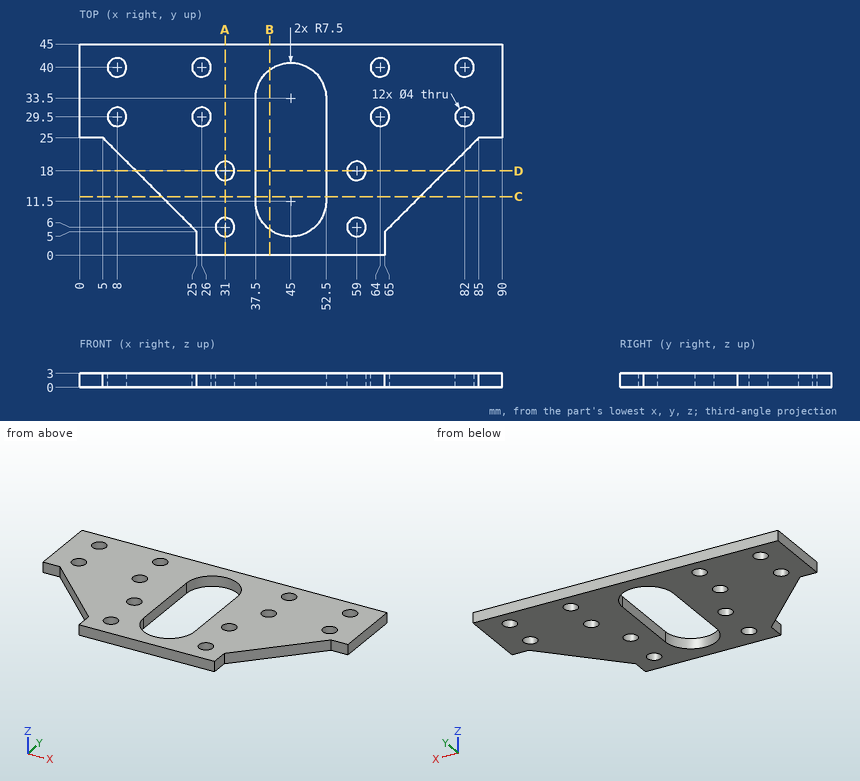
Part print with two shaded views. Sizes in mm from the minimum x, y, z corner. Coordinates: 2 decimals unless noted, no trailing zeros. Order: outer loops, then holes, each group sorted by start corner. A loop starts at its lowest first (then second) coordinate and runs counter-clockwise, first axis right, second up. Notation, with made-up numbers: (-21, 76.5) - (5, 76.5) arc R8 ccw to (5, 88.5) - close; hole circle Ø2 at (42, 74). An arc over 180 degrees is marked (long way). Answer in a Markdown table with one row per item.
1. Slice it at D-D, the plane y = 18. List the corners of the cut face in (x, z).
Answer:
| item | result |
|---|---|
| outline | (12, 0) - (29, 0) - (29, 3) - (12, 3) - close; (33, 0) - (37.5, 0) - (37.5, 3) - (33, 3) - close; (52.5, 0) - (57, 0) - (57, 3) - (52.5, 3) - close; (61, 0) - (78, 0) - (78, 3) - (61, 3) - close |
2. Drill centre lines: L1, parallel to X at y = 26.5, z = 0.55; L2, parallel to X at y = 30, z = 1.95; L3, parallel to Y at x = 24.5, z = 0.7. Where is each one in solid material? Low to high. Write a range as from..to.
Answer:
| item | result |
|---|---|
| L1 | 0..37.5, 52.5..90 |
| L2 | 0..6.06, 9.94..24.06, 27.94..37.5, 52.5..62.06, 65.94..80.06, 83.94..90 |
| L3 | 5.5..28.18, 30.82..38.68, 41.32..45 |
3. Slice it at B-B, the plane x = 40.5. List the corners of the cut face in (y, z).
Answer:
| item | result |
|---|---|
| outline | (0, 0) - (5.5, 0) - (5.5, 3) - (0, 3) - close; (39.5, 0) - (45, 0) - (45, 3) - (39.5, 3) - close |
4. Flat gauge pins, fed straight in: P1, Ø1.5, axis at y = 18, z = 2, coming from the -X side; P2, Ø5, axis at x = 64, y = 40, coming from the -Z side; P3, Ø1.5, axis at y = 2.5, z = 1.5, coming from the -X side; P4, Ø1.5, axis at y = 3, z = 1, coming from the +X side. Where does each tip first touch, or does it go through?
Answer:
| item | result |
|---|---|
| P1 | x = 11.25 |
| P2 | z = 0 |
| P3 | x = 25 |
| P4 | x = 65 |
5. Slice it at A-A, the plane x = 31. List the corners of the cut face in (y, z).
Answer:
| item | result |
|---|---|
| outline | (0, 0) - (4, 0) - (4, 3) - (0, 3) - close; (8, 0) - (16, 0) - (16, 3) - (8, 3) - close; (20, 0) - (45, 0) - (45, 3) - (20, 3) - close |
6. Slice it at C-C, the plane y = 12.5. List the corners of the cut face in (x, z), then the cut area to 3 significant figures.
Answer:
| item | result |
|---|---|
| outline | (17.5, 0) - (37.5, 0) - (37.5, 3) - (17.5, 3) - close; (52.5, 0) - (72.5, 0) - (72.5, 3) - (52.5, 3) - close |
| area | 120 mm² |
